```python
from build123d import *

# Parameters (mm, degrees)
SKETCH_1_R      = 1.5
EXTRUDE_1_DEPTH = 4


with BuildPart() as part:
    # 草图1 → 凸台-拉伸1 (new body)
    with BuildSketch(Plane.XY):
        with BuildLine():
            add(Edge.make_bspline(
                [(0, 10), (52.11400991, 10.48088872), (106.792215868, 14.291406746), (151.130268959, 38.519700222)],
                knots=[0.172138622, 0.172138622, 0.172138622, 0.172138622, 0.832549304, 0.832549304, 0.832549304, 0.832549304], degree=3))
            add(Edge.make_bspline(
                [(-0.183054557, 9.998324411), (-0.122039901, 9.998878394), (-0.061021708, 9.999436914), (0, 10)],
                knots=[0.17136533, 0.17136533, 0.17136533, 0.17136533, 0.172138622, 0.172138622, 0.172138622, 0.172138622], degree=3))
            add(Edge.make_bspline(
                [(-39.962254298, 9.999928763), (-27.025718651, 9.975441168), (-13.691052102, 9.875678503), (-0.183054557, 9.998324411)],
                knots=[0.000166511, 0.000166511, 0.000166511, 0.000166511, 0.17136533, 0.17136533, 0.17136533, 0.17136533], degree=3))
            ThreePointArc((-39.962254298, 9.999928763), (-39.981127115, 9.999982191), (-40, 10))
            ThreePointArc((-40, 10), (-50, 0), (-40, -10))
            add(Edge.make_bspline(
                [(-40, -10), (-26.629572895, -10.441521612), (-13.296239562, -10.441521612), (0, -10)],
                knots=[0, 0, 0, 0, 0.198467229, 0.198467229, 0.198467229, 0.198467229], degree=3))
            add(Edge.make_bspline(
                [(0, -10), (0.224885721, -9.992532332), (0.449760832, -9.984938359), (0.674625331, -9.977218082)],
                knots=[0.198467229, 0.198467229, 0.198467229, 0.198467229, 0.201824001, 0.201824001, 0.201824001, 0.201824001], degree=3))
            add(Edge.make_bspline(
                [(0.674625331, -9.977218082), (30.932305536, -8.938380612), (60.997855132, -5.612641251), (90.871274119, 0)],
                knots=[0.201824001, 0.201824001, 0.201824001, 0.201824001, 0.653509958, 0.653509958, 0.653509958, 0.653509958], degree=3))
            Line((90.871274119, 0), (163.684000861, 17.723388911))
            ThreePointArc((163.684000861, 17.723388911), (171.094194245, 33.297976406), (155.725788693, 41.126823857))
            ThreePointArc((155.725788693, 41.126823857), (153.287141392, 40.071601234), (151.130268959, 38.519700222))
        make_face()
        with Locations((-40, 0)):
            Circle(SKETCH_1_R, mode=Mode.SUBTRACT)
        Circle(SKETCH_1_R, mode=Mode.SUBTRACT)
    extrude(amount=EXTRUDE_1_DEPTH)


solid = part.part
```
Here's how the part is built. I have some questions about the finished solid (model axes, mm). Coordinates: 2 decimals unless noted, no trailing zeros. Write each loop counter-clockwise with the first axis right and the second up, starting at its lowest first coordinate (ties: lowest second). Pieces come first, ordered by that corner, then holes. Notation, with made-up numbers: M -13,27.25 L 3,27.25 A11 ccw 3,41.25 Z; hole C -6.75,-36 d1. An arc over 180 degrees is marked long. Answer as CSV lines item,"result". Start each with the question number.
Q1. I need wall thicknesses on probe 1 along Y at (x, z) = (0, 2.35); probe 2 along Y at (x, z) = (-24.5, 0.6); probe 3 along X at (y, z) = (39.5, 1). Which ranges of each line are inside material? Lowest first, please. Write a range as [from, to].
Q2. Suppose I cut it at B-B, the plane y = 5.5. List the corners of the cut face in (x, z) for me, then the cut area to 3 significant figures.
Q3. Suppose I cut it at A-A, the plane z = 2.05. State how many separate pieces and enclosed holes the cut face has, then the cut area to 3 significant figures.
Q4. Will these pins go through, and if not, where does the flat tip stop? pin 1 Ø2 at (x, z) = (39, 1) entering from +Y; pin 2 Ø1.8 at (x, y) = (-40, 0) entering from +Z.
Entries:
1,probe 1,"y = [-10, -1.5], [1.5, 10]"
1,probe 2,"y = [-10.31, 9.95]"
1,probe 3,"x = [152.37, 166.4]"
2,outline,"M -48.35,0 L 113.47,0 L 113.47,4 L -48.35,4 Z"
2,area,"647 mm²"
3,separate pieces,"1"
3,enclosed holes,"2"
3,area,"4,230 mm²"
4,pin 1,"stops at y = 11.29"
4,pin 2,"passes through"
